Here's how the part is built. I have some questions about the finished solid (model axes, mm). A direction names the side the tool comes from. Coordinates: 2 decimals unless noted, no trailing zeros. Write each loop counter-clockwise with the first axis right and the second up, starting at its lowest first coordinate (ties: lowest second). Pieces come first, ordered by that corner, then holes. Notation, with made-up numbers: M -2,19 L 51,19 A19 ccw 51,48 Z; hole C 7,-9.5 d4. An arc over 180 degrees is marked long. Write each question's results on one line, items separated by ' | '. Start each with the question number.
from build123d import *

# Parameters (mm, degrees)
F0_W     = 34.8
F0_H     = 4.6
F1_DEPTH = 34.6
F0_W_2   = 4.2
F0_H_2   = 0.8
F2_DEPTH = 29.8


with BuildPart() as f1:
    # F0 (on Front) → F1 (new body, symmetric)
    with BuildSketch(Plane.XZ):
        with Locations((-3.756187, 0.384168)):
            Rectangle(F0_W, F0_H)
    extrude(amount=F1_DEPTH, both=True)

    # F0 (on Front) → F2 (join, symmetric)
    with BuildSketch(Plane.XZ):
        Polygon((13.643813, 3.684168), (-21.156187, 3.684168), (-21.156187, 2.684168), (13.643813, 2.684168), (13.643813, 2.884168), align=None)
        Polygon((13.643813, -1.915832), (-21.156187, -1.915832), (-21.156187, -2.915832), (13.643813, -2.915832), (13.643813, -2.115832), align=None)
        with Locations((15.743813, -2.515832)):
            Rectangle(F0_W_2, F0_H_2)
        with Locations((15.743813, 3.284168)):
            Rectangle(F0_W_2, F0_H_2)
    extrude(amount=F2_DEPTH, both=True)


solid = f1.part
1) For faces 4 (the flat face through (16, 0, 2.884)), 5 (the flat face through (-4, -32, 2.684)), 6 (the flat face through (-4, 32, -1.916)), 7 (the flat face through (-4, -32, -1.916)), 8 (the flat face through (-21.156, 0, 0)), which set-ups out of +Z, -Z, +X, -X, +Y, -Y let a thin tool reach every point of the face, with its end or its side?
2) For pin 1 Ø4 at (x, y) = (-3.5, 32) entering from +Z; pin 2 Ø4 at (x, y) = (-9.5, -32) entering from -Z; pin 3 Ø1.1 at (x, z) = (3.5, -2.5) entering from -Y; pin 4 Ø0.8 at (x, z) = (7.5, 3) entering from +Y, each with a flat end and sliding along its axis, tell me the tip position at first contact or that it passes through.
3) I want a section at C-C, the plane z = 1. Write out the boundary of the cut face in (x, y).
4) I want a section at B-B, the plane x = 10. Write out the boundary of the cut face in (y, z), then the cut area to 3 significant figures.
5) Please list where these lines run through material, in increasing order: line 1 (Z direction, x = 16, y = 23); line 2 (X direction, y = 24, z = 1.25); line 3 (Z direction, x = 9.5, y = 32). Write a range as [from, to].
6) We'd pull the mould along Z, two halves only. Please class faces 1 (the flat face through (-2, 0, -2.916)), 2 (the flat face through (16, 0, -2.116)), 3 (the flat face through (-4, 32, 2.684)): pulls with the +Z half, pulls with the -Z half, needs draft (parallel to the pull), parting line crosses it, or undercut.
7) I want a section at A-A, the plane y = -10.5. Write out the boundary of the cut face in (x, z).
Output:
1) face 4: +X, +Y, -Y | face 5: +Z, +X, -X, -Y | face 6: -Z, +X, -X, +Y | face 7: -Z, +X, -X, -Y | face 8: +Z, -Z, -X, +Y, -Y
2) pin 1: stops at z = 2.68 | pin 2: stops at z = -1.92 | pin 3: stops at y = -29.8 | pin 4: stops at y = 34.6
3) outline: M -21.16,-34.6 L 13.64,-34.6 L 13.64,34.6 L -21.16,34.6 Z
4) outline: M -34.6,-1.92 L -29.8,-1.92 L -29.8,-2.92 L 29.8,-2.92 L 29.8,-1.92 L 34.6,-1.92 L 34.6,2.68 L 29.8,2.68 L 29.8,3.68 L -29.8,3.68 L -29.8,2.68 L -34.6,2.68 Z | area: 438 mm2
5) line 1: z = [-2.92, -2.12], [2.88, 3.68] | line 2: x = [-21.16, 13.64] | line 3: z = [-1.92, 2.68]
6) face 1: pulls with the -Z half | face 2: undercut | face 3: pulls with the +Z half
7) outline: M -21.16,-2.92 L 17.84,-2.92 L 17.84,-2.12 L 13.64,-2.12 L 13.64,2.88 L 17.84,2.88 L 17.84,3.68 L -21.16,3.68 Z
